```python
from build123d import *

# Parameters (mm, degrees)
SKETCH1_W                  = 92.075
SKETCH1_H                  = 63.5
SKETCH1_R                  = 3.937
EXTRUDE1_DEPTH             = 3.96875
SKETCH2_W                  = 50.8
SKETCH2_H                  = 2.38125
EXTRUDE2_DEPTH             = 100.80625
FILLET1_R                  = 25.4
EXTRUDE3_REACH             = 117.28
SKETCH3_R                  = 6.35
EXTRUDE3_DIRECTION_2_REACH = 117.28
SKETCH4_R                  = 50.8
EXTRUDE4_DEPTH             = 15.875
FILLET2_R                  = 3.175
FILLET3_R                  = 3.175


with BuildPart() as part:
    # Sketch1 → Extrude1 (new body)
    with BuildSketch(Plane(origin=(0, 0, 0), x_dir=(1, 0, 0), z_dir=(0, 1, 0))):
        Rectangle(SKETCH1_W, SKETCH1_H)
        with Locations(Location((-37.30625, 22.225, 0), (0, 0, 270))):
            Circle(SKETCH1_R, mode=Mode.SUBTRACT)
        with Locations(Location((-37.30625, -22.225, 0), (0, 0, 270))):
            Circle(SKETCH1_R, mode=Mode.SUBTRACT)
        with Locations(Location((37.30625, -22.225, 0), (0, 0, 270))):
            Circle(SKETCH1_R, mode=Mode.SUBTRACT)
        with Locations(Location((37.30625, 22.225, 0), (0, 0, 270))):
            Circle(SKETCH1_R, mode=Mode.SUBTRACT)
    extrude(amount=EXTRUDE1_DEPTH)

    # Sketch2 → Extrude2 (add)
    with BuildSketch(Plane(origin=(0, 0, 0), x_dir=(-1, 0, 0), z_dir=(0, 1, 0))):
        with Locations((0, 18.653125)):
            Rectangle(SKETCH2_W, SKETCH2_H)
        with Locations((0, -18.653125)):
            Rectangle(SKETCH2_W, SKETCH2_H)
    extrude(amount=-EXTRUDE2_DEPTH)

    # Fillet1
    fillet1_edges = [part.edges().sort_by_distance(p)[0] for p in [
        (-25.4, -100.80625, 18.653125),
        (-25.4, -100.80625, -18.653125),
        (25.4, -100.80625, -18.653125),
        (25.4, -100.80625, 18.653125),
    ]]
    fillet(fillet1_edges, radius=FILLET1_R - 0.0001)  # a hair under: the kernel refuses the full size

    # Sketch3 → Extrude3 (add, up to next)
    with BuildSketch(Plane.XY, mode=Mode.PRIVATE) as extrude3_sk1:
        with Locations((0, -75.40625)):
            Circle(SKETCH3_R)
    extrude3_tool1 = extrude(extrude3_sk1.sketch, amount=EXTRUDE3_REACH, mode=Mode.PRIVATE) - part.part
    add(extrude3_tool1.solids().sort_by_distance((0, -75.40625, 0))[0])

    # Sketch3 → Extrude3 direction 2 (add, up to next)
    with BuildSketch(Plane.XY, mode=Mode.PRIVATE) as extrude3_direction_2_sk1:
        with Locations((0, -75.40625)):
            Circle(SKETCH3_R)
    extrude3_direction_2_tool1 = extrude(extrude3_direction_2_sk1.sketch, amount=-EXTRUDE3_DIRECTION_2_REACH, mode=Mode.PRIVATE) - part.part
    add(extrude3_direction_2_tool1.solids().sort_by_distance((0, -75.40625, 0))[0])

    # Sketch4 → Extrude4 (add, symmetric)
    with BuildSketch(Plane.XY):
        with Locations((0, -75.40625)):
            Circle(SKETCH4_R)
    extrude(amount=EXTRUDE4_DEPTH, both=True)

    # Fillet2
    fillet2_edges = [part.edges().sort_by_distance(p)[0] for p in [
        (-50.8, -75.40625, -15.875),
        (-50.8, -75.40625, 15.875),
    ]]
    fillet(fillet2_edges, radius=FILLET2_R)

    # Fillet3
    fillet3_edges = [part.edges().sort_by_distance(p)[0] for p in [
        (-46.0375, 1.984375, -31.75),
        (46.0375, 1.984375, -31.75),
        (46.0375, 1.984375, 31.75),
        (-46.0375, 1.984375, 31.75),
    ]]
    fillet(fillet3_edges, radius=FILLET3_R)


solid = part.part
```
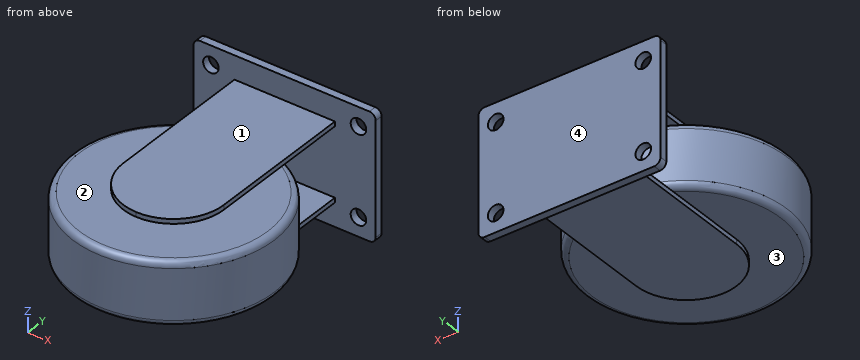
Input: part model. Units: mm. Frame: model coordinates. Face numbers are marked on the shaded views. Round coordinates to 2 decimals unless told otherwise and drop trailing zeros. Loops run counter-clockwise (first coordinate to the right, second up) from the corner with the lowest first, then second, coordinate; pieces in that order, holes last. Notation, with made-up numbers: (-2.5, 40.5) -> (23.5, 40.5) arc R8 cw to (23.5, 46.5) -> close; hole circle Ø2 at (70.5, -38.75). An arc over 180 degrees is marked (long way). Use one line per item in the form item = value. Start each with the question number.
Item 1: Section query A-A on z = 23. Return the cut outline in (x, y).
Item 2: Section query B-B on z = 1. Return the cut outline in (x, y).
Item 3: Section query C-C on x = -39.5. Count the separate pieces of the cut face and the enclosed holes in it, then the cut area to 3 significant figures.
Item 4: Material intervals for L1, parallel to Z at x = 24.5, y = -53 (1 decimal); L2, parallel to Z at x = 14.5, y = -3.5; L3, parallel to Z at x = -32, y = -85 (3 decimals), sorted ascending. Write a range as from..to.
Item 5: Contact query for flat-ended pins moving along their axis: pin 1 Ø3 at (x, z) = (31, 14.5) entering from -Y; pin 2 Ø15 at (x, y) = (-12, -73.5) entering from +Z; pin 3 Ø3 at (y, z) = (1.5, -1) entering from -X. Output: stop coordinate, or through.
Item 6: Mould query, pull axis Z, two halves, no side actions, for the marked faces 1, 2, 3 and 4. Classes: pulls with the +Z half, pulls with the -Z half, needs draft (parallel to the pull), parting line crosses it, or undercut.
Ans:
q1.outline = (-46.04, 0) -> (-41.17, 0) -> (-41.17, 3.97) -> (-46.04, 3.97) -> close; (-33.45, 0) -> (33.45, 0) -> (33.45, 3.97) -> (-33.45, 3.97) -> close; (41.17, 0) -> (46.04, 0) -> (46.04, 3.97) -> (41.17, 3.97) -> close
q2.outline = circle Ø101.6 at (0, -75.41); (-46.04, 0) -> (46.04, 0) -> (46.04, 3.97) -> (-46.04, 3.97) -> close
q3.separate_pieces = 4
q3.enclosed_holes = 0
q3.area = 2,210 mm^2
q4.L1 = -19.8..-17.5, -15.9..15.9, 17.5..19.8
q4.L2 = -19.84..-17.46, 17.46..19.84
q4.L3 = -15.875..15.875
q5.pin_1 = -116.4
q5.pin_2 = 19.84
q5.pin_3 = -46.04
q6.face_1 = pulls with the +Z half
q6.face_2 = undercut
q6.face_3 = undercut
q6.face_4 = needs draft
